Geometry: see drawing. Coordinates: mm, zero at the bounding-box minimum. A direction names the side the tool comes from. Coordinates: 2 decimals unless noted, no trailing zeros. Loops run counter-clockwise (first coordinate to the right, second up) from the corner with the lowest first, then second, coordinate; pieces in that order, holes last.
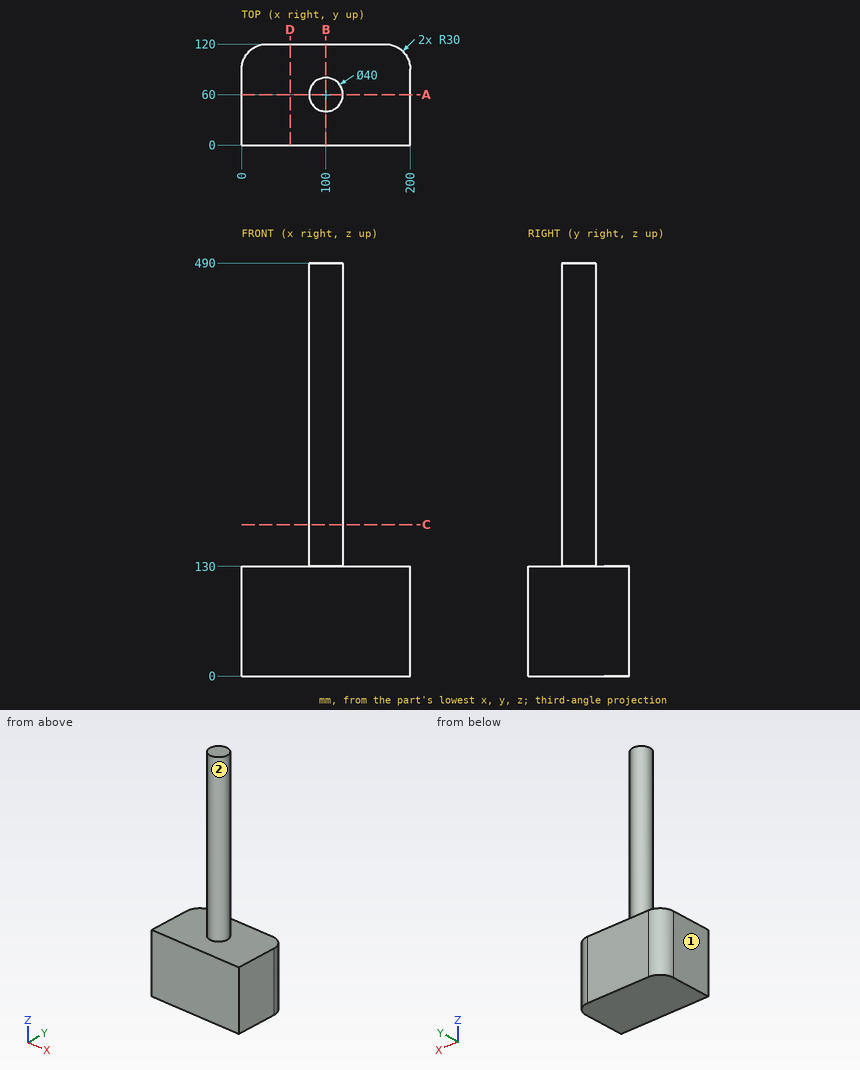
Item 1: Section query D-D (x = 57.5). Output: boundary loops of the cut face in (y, z).
Result:
outline: (0, 0) - (120, 0) - (120, 130) - (0, 130) - close
Item 2: Section query B-B (x = 100). Output: boundary loops of the cut face in (y, z).
Result:
outline: (0, 0) - (120, 0) - (120, 130) - (80, 130) - (80, 490) - (40, 490) - (40, 130) - (0, 130) - close
Item 3: Line query: L1, parallel to Z at x = 10.5, y = 7; L2, parallel to Y at x = 181, z = 123; L3, parallel to Y at x = 177, z = 30. Output: solid intervals per line, ascending.
Result:
L1: z = 0 to 130
L2: y = 0 to 117.91
L3: y = 0 to 119.17
Item 4: Section query C-C (z = 179.5). Output: boundary loops of the cut face in (x, y), then the cut area to 3 significant figures.
Result:
outline: circle Ø40 at (100, 60)
area: 1,260 mm2
Item 5: Contact query for flat-ended pins moving along their axis: P1, Ø10, axis at x = 152.5, z = 136.5, coming from the +Y side; P2, Ø10, axis at x = 172, y = 85.5, coming from the +Z side. Output: stop coordinate, or through.
Result:
P1: passes through
P2: stops at z = 130
Item 6: Section query A-A (y = 60). Output: boundary loops of the cut face in (x, z), then the cut area to 3 significant figures.
Result:
outline: (0, 0) - (200, 0) - (200, 130) - (120, 130) - (120, 490) - (80, 490) - (80, 130) - (0, 130) - close
area: 40,400 mm2
Item 7: Reachability of the marked faces 1 and 2 from +Z, -Z, +X, -X, +Y, -Y: full face, straight path, thin tool, end or side. Return the list, or none.
Result:
face 1: +Z, -Z, -X, +Y, -Y
face 2: +Z
